Can you work these out from the model? Positions are in its coordinate system, mm. Face numbers are marked on the shaded views. Round coordinates to 2 decimals unless told otherwise and drop trailing zeros. Loops run counter-clockwise (first coordinate to the right, second up) from the corner with the lowest first, then second, coordinate; pieces in that order, holes last. Notation, with made-up numbers: (59.25, -40) - (87.25, -40) arc R28 ccw to (87.25, -7) - close; hole circle Ø10 at (82, -1.5). An arc over 180 degrees is marked (long way). Answer as CSV lines item,"result".
```python
from build123d import *

# Parameters (mm, degrees)
F1_DEPTH = 0.11
F2_W     = 0.11
F2_H     = 90
F3_DEPTH = 40
F4_W     = 0.11
F4_H     = 90
F5_DEPTH = 5
F6_W     = 54.38837
F6_H     = 0.11
F7_DEPTH = 5


with BuildPart() as f1:
    # F0 (on Front) → F1 (new body)
    with BuildSketch(Plane.XZ):
        Polygon((12.805815, 12.805815), (0, 0), (0, -90), (7.5, -90), (7.5, -25), (72.5, -25), (72.5, -90), (80, -90), (80, 0), (67.194185, 12.805815), align=None)
        Polygon((16.2438, 5), (36.2438, 5), (36.2438, -15), (5, -15), (5, -6.2438), align=None, mode=Mode.SUBTRACT)
        Polygon((42.101238, -15), (42.101238, 5), (62.101238, 5), (75, -7.898762), (75, -15), align=None, mode=Mode.SUBTRACT)
    extrude(amount=F1_DEPTH)

    # F2 (on face) → F3 (join)
    with BuildSketch(Plane(origin=(0, 0, 0), x_dir=(-1, 0, 0), z_dir=(0, 1, 0))):
        with Locations((-0.055, -45)):
            Rectangle(F2_W, F2_H)
    extrude(amount=F3_DEPTH)

    # F4 (on face) → F5 (join)
    with BuildSketch(Plane.YZ.offset(0.11)):
        with Locations((39.945, -45)):
            Rectangle(F4_W, F4_H)
    extrude(amount=F5_DEPTH)

    # F6 (on face) → F7 (join)
    with BuildSketch(Plane(origin=(0, 0, 0), x_dir=(-1, 0, 0), z_dir=(0, 1, 0))):
        with Locations((-40, 12.750815)):
            Rectangle(F6_W, F6_H)
    extrude(amount=F7_DEPTH)


solid = f1.part
```
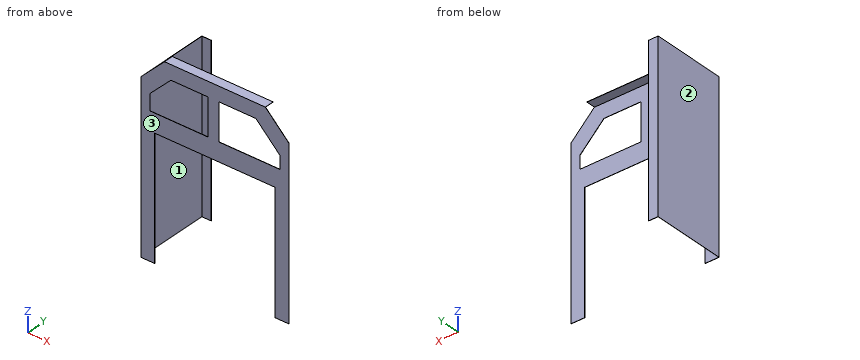
Q1. Imagine slicing it at B-B (x = 52). Write out the boundary of the cut face in (y, z), then the cut area to 3 significant figures.
Checks:
outline,"(-0.11, -25) - (0, -25) - (0, -15) - (-0.11, -15) - close; (-0.11, 5) - (0, 5) - (0, 12.7) - (5, 12.7) - (5, 12.81) - (-0.11, 12.81) - close"
area,"2.51 mm²"
Q2. We'd pull the mould along Y, two halves only. Please class the marked faces 1, 2 and 3: pulls with the +Y half, pulls with the -Y half, needs draft (parallel to the pull), parting line crosses it, or undercut.
Checks:
face 1,"undercut"
face 2,"needs draft"
face 3,"pulls with the -Y half"
Q3. I'm going to push flat-ended pins straight in: pin 1 Ø4 at (x, y) = (1.5, 20.5) entering from +Z; pin 2 Ø12 at (x, z) = (60, -23.5) entering from +Y; pin 3 Ø4 at (x, y) = (40, 3.5) entering from -Z. Where does each tip first touch, or does it pass through?
Checks:
pin 1,"z = 0"
pin 2,"y = 0"
pin 3,"z = 12.7"
Q4. Imagine slicing it at C-C (z = -11). Write out the boundary of the cut face in (x, y), then the cut area to 3 significant figures.
Checks:
outline,"(0, -0.11) - (5, -0.11) - (5, 0) - (0.11, 0) - (0.11, 39.89) - (5.11, 39.89) - (5.11, 40) - (0, 40) - close; (36.24, -0.11) - (42.1, -0.11) - (42.1, 0) - (36.24, 0) - close; (75, -0.11) - (80, -0.11) - (80, 0) - (75, 0) - close"
area,"6.69 mm²"
Q5. Imagine slicing it at D-D (z = -22). Write out the boundary of the cut face in (x, y), then the cut area to 4 significant figures.
Checks:
outline,"(0, -0.11) - (80, -0.11) - (80, 0) - (0.11, 0) - (0.11, 39.89) - (5.11, 39.89) - (5.11, 40) - (0, 40) - close"
area,"13.75 mm²"
Q6. Imagine slicing it at A-A (z = -62). Write out the boundary of the cut face in (x, y).
Checks:
outline,"(0, -0.11) - (7.5, -0.11) - (7.5, 0) - (0.11, 0) - (0.11, 39.89) - (5.11, 39.89) - (5.11, 40) - (0, 40) - close; (72.5, -0.11) - (80, -0.11) - (80, 0) - (72.5, 0) - close"
